Autodesk Inventor part; units mm, degrees
ref_plane "YZ Plane" through (0, 0, 0) normal (1, 0, 0) x (0, 1, 0)
ref_plane "XZ Plane" through (0, 0, 0) normal (0, 1, 0) x (-1, 0, 0)
ref_plane "XY Plane" through (0, 0, 0) normal (0, 0, 1) x (1, 0, 0)
sketch "スケッチ1" plane through (0, 0, 0) normal (0, 0, 1) x (1, 0, 0)
  circle A0 centre (-7.5, 0) radius 1.25
  circle A1 centre (7.5, 0) radius 1.25
  line L0 (-14, -10.5) -> (-5.5, -10.5) construction
  line L1 (22, 10) -> (-22, 10)
  arc A2 (-18.7483, 4) -> (-17.2517, 4) centre (-18, 2.7) ccw construction
  arc A3 (17.2517, 4) -> (18.7483, 4) centre (18, 2.7) ccw construction
  line L2 (-22, 10) -> (-22, 4)
  line L3 (-22, 4) -> (-18.7483, 4)
  line L4 (-14, 4) -> (-14, 0)
  line L5 (22, 10) -> (22, 4)
  line L6 (22, 4) -> (18.7483, 4)
  line L7 (14, 4) -> (14, 0)
  arc A4 (-17.2517, 4) -> (-18.7483, 4) centre (-18, 2.7) ccw
  line L8 (-18.7483, 4) -> (-17.2517, 4) construction
  line L9 (-17.2517, 4) -> (-14, 4)
  arc A5 (18.7483, 4) -> (17.2517, 4) centre (18, 2.7) ccw
  line L10 (18.7483, 4) -> (17.2517, 4) construction
  line L11 (17.2517, 4) -> (14, 4)
  arc A6 (-14, 0) -> (-11.8293, -4.8484) centre (-7.5, 0) ccw
  arc A7 (11.8293, -4.8484) -> (14, 0) centre (7.5, 0) ccw
  line L12 (-11.8293, -4.8484) -> (-5.5, -10.5)
  line L13 (11.8293, -4.8484) -> (5.5, -10.5)
  line L14 (-14, 0) -> (-14, -10.5) construction
  line L15 (-5.5, -10.5) -> (5.5, -10.5)
  line L16 (5.5, -10.5) -> (14, -10.5) construction
  line L17 (14, 0) -> (14, -10.5) construction
  point P0 (0, 0)
  dimension "d0" = 2.5
  dimension "d1" = 2.5
  dimension "d2" = 15
  dimension "d3" = 7.5
  dimension "d8" = 10.5
  dimension "d9" = 10
  dimension "d15" = 3
  dimension "d16" = 3
  dimension "d21" = 6.5
  dimension "d22" = 6.5
  dimension "d23" = 10.5
  dimension "d24" = 6
  dimension "d25" = 6
  dimension "d26" = 8
  dimension "d27" = 8
  dimension "d28" = 1.3
  dimension "d29" = 1.3
  dimension "d30" = 4
  dimension "d31" = 4
  dimension "d34" = 11
  dimension "d35" = 5.5
extrude "押し出し1" add sketch "スケッチ1" along normal blind 6
properties part number "ベルト固定_アルミ"
Geometry: final body of the model. Coordinates: model frame, mm. A direction names the side the tool comes from. Round coordinates to 2 decimals unless told otherwise and drop trailing zeros. Order: outer loops, then holes, each group sorted by start corner. A loop starts at its lowest first (then second) coordinate and runs counter-clockwise, first axis right, second up.
Q1. Mould query, pull axis Y, two halves, no side actions, for faces 4 (the face through (0, -10.5, 3)), 5 (the face through (0, 10, 3)), 6 (the face through (-8.75, -0.05, 2.96)), 7 (the face through (0, 2, 6)). Classes: released by +Y, released by -Y, zero draft, split by the parting line, or undercut.
Result sheet:
face 4: released by -Y
face 5: released by +Y
face 6: undercut
face 7: zero draft
Q2. Section C-C, the plane x = 18. Output: boundary loops of the cut face in (y, z).
Result sheet:
outline: (4.2, 0) - (10, 0) - (10, 6) - (4.2, 6) - close
Q3. Section D-D, the plane y = -3. Output: boundary loops of the cut face in (x, z).
Result sheet:
outline: (-13.27, 0) - (13.27, 0) - (13.27, 6) - (-13.27, 6) - close
Q4. Section B-B, the plane x = 7.5. Output: boundary loops of the cut face in (y, z).
Result sheet:
outline: (-8.71, 0) - (-1.25, 0) - (-1.25, 6) - (-8.71, 6) - close; (1.25, 0) - (10, 0) - (10, 6) - (1.25, 6) - close
Q5. Access query for faces 1 (the face through (18, 4.2, 3)), 2 (the face through (-16, 4, 3)), 3 (the face through (20, 4, 3)). Directions: +Z, -Z, +X, -X, +Y, -Y. A direction counts if a zero-diameter tool reaches every point of the face in a straight line with its end or side. Return the directions, or none.
Result sheet:
face 1: +Z, -Z, -Y
face 2: +Z, -Z, -X, -Y
face 3: +Z, -Z, +X, -Y
Q6. Pin query (flat end, axial travel): pin 1 (3.5 mm diameter, centred on x = -16, z = 3, fed in from -Y); pin 2 (1 mm diameter, centred on y = 1.5, z = 5, fed in from -X). Return the tip coordinate at first contact, or that it passes through.
Result sheet:
pin 1: stops at y = 4
pin 2: stops at x = -14
Q7. Section A-A, the plane z = 3.45. Output: boundary loops of the cut face in (x, y), and give its area (3 significant figures).
Result sheet:
outline: (-22, 4) - (-18.75, 4) arc R1.5 cw to (-17.25, 4) - (-14, 4) - (-14, 0) arc R6.5 ccw to (-11.83, -4.85) - (-5.5, -10.5) - (5.5, -10.5) - (11.83, -4.85) arc R6.5 ccw to (14, 0) - (14, 4) - (17.25, 4) arc R1.5 cw to (18.75, 4) - (22, 4) - (22, 10) - (-22, 10) - close; hole circle Ø2.5 at (-7.5, 0); hole circle Ø2.5 at (7.5, 0)
area: 593 mm2
Q8. Material intervals for probe 1 along X at (y, z) = (-0.25, 0.95); probe 2 along X at (y, z) = (-0.75, 3.5); probe 3 along Y at (x, z) = (-20, 0.75), sorted ascending.
Result sheet:
probe 1: x = -14 to -8.72, -6.28 to 6.28, 8.72 to 14
probe 2: x = -13.96 to -8.5, -6.5 to 6.5, 8.5 to 13.96
probe 3: y = 4 to 10
